Work out the finished part from the listing and answer in its coordinate system (mm). Face numbers are marked on the shaded views. A direction names the side the tool comes from. Round coordinates to 2 decimals unless told otherwise and drop trailing zeros. Write each loop counter-clockwise with the first axis right and the second up, starting at its lowest first coordinate (ties: lowest second). Pieces come first, ordered by that corner, then holes. Notation, with made-up numbers: (87, 16.5) -> (94, 16.5) arc R32 ccw to (94, 52.5) -> close; hole circle Ø9 at (74, -34.75). An arc over 180 degrees is marked (long way). One line per item, written item: value.
```python
from build123d import *

# Parameters (mm, degrees)
SKETCH2_W               = 90
SKETCH2_H               = 90
BOSS_EXTRUDE1_DEPTH     = 103
SKETCH4_W               = 24
SKETCH4_H               = 25
SKETCH4_W_2             = 40
SKETCH4_H_2             = 17.5
SKETCH4_W_3             = 3
SKETCH4_H_3             = 4
SKETCH5_R               = 10
CUT_EXTRUDE1_DEPTH      = 46
CUT_EXTRUDE1_DEPTH_BACK = 46
SKETCH6_W               = 80.499612835
SKETCH6_H               = 43.101198191
CUT_EXTRUDE2_DEPTH      = 46
CUT_EXTRUDE2_DEPTH_BACK = 46
CUT_EXTRUDE3_DEPTH      = 103
CUT_EXTRUDE4_REACH      = 92
SKETCH10_R              = 1.75
FILLET1_R               = 1


with BuildPart() as part:
    # Sketch2 → Boss-Extrude1 (new body)
    with BuildSketch(Plane.XY):
        Rectangle(SKETCH2_W, SKETCH2_H)
    extrude(amount=BOSS_EXTRUDE1_DEPTH)

    # Sketch4 → Cut-Revolve2 (revolve, cut)
    with BuildSketch(Plane(origin=(0, 0, 0), x_dir=(1, 0, 0), z_dir=(0, 1, 0))):
        with Locations((12, -12.5)):
            Rectangle(SKETCH4_W, SKETCH4_H)
        Polygon((0, -25), (0, -39.420654857), (24, -25), align=None)
        with Locations((50, -8.75)):
            Rectangle(SKETCH4_W_2, SKETCH4_H_2)
        with Locations((28.5, -4.5)):
            Rectangle(SKETCH4_W_3, SKETCH4_H_3)
    revolve(axis=Axis((0, 0, 0), (0, 0, 1)), mode=Mode.SUBTRACT)

    # Sketch5 → Cut-Extrude1 (cut, two sides)
    with BuildSketch(Plane(origin=(0, 0, 0), x_dir=(0, 0, -1), z_dir=(1, 0, 0))) as cut_extrude1_sk:
        with Locations((-77.5, 0)):
            Circle(SKETCH5_R)
    extrude(amount=CUT_EXTRUDE1_DEPTH, mode=Mode.SUBTRACT)
    extrude(cut_extrude1_sk.sketch, amount=-CUT_EXTRUDE1_DEPTH_BACK, mode=Mode.SUBTRACT)

    # Sketch6 → Cut-Revolve3 (revolve, cut)
    with BuildSketch(Plane(origin=(0, 0, 0), x_dir=(0, 0, -1), z_dir=(1, 0, 0))):
        with Locations((-94.419607416, 51.550599096)):
            Rectangle(SKETCH6_W, SKETCH6_H)
    revolve(axis=Axis((0, 0, 0), (0, 0, 1)), mode=Mode.SUBTRACT)

    # Sketch7 → Cut-Extrude2 (cut, two sides)
    with BuildSketch(Plane(origin=(0, 0, 0), x_dir=(0, 0, -1), z_dir=(1, 0, 0))) as cut_extrude2_sk:
        with BuildLine():
            Line((-103, 30), (-103, 0))
            ThreePointArc((-103, 0), (-95.748626332, 19.557607216), (-77.5, 29.6605799))
            Line((-77.5, 29.6605799), (-77.5, 30))
            Line((-77.5, 30), (-103, 30))
        make_face()
        with BuildLine():
            ThreePointArc((-77.5, -29.6605799), (-95.748626332, -19.557607216), (-103, 0))
            Line((-103, 0), (-103, -30))
            Line((-103, -30), (-77.5, -30))
            Line((-77.5, -30), (-77.5, -29.6605799))
        make_face()
    extrude(amount=CUT_EXTRUDE2_DEPTH, mode=Mode.SUBTRACT)
    extrude(cut_extrude2_sk.sketch, amount=-CUT_EXTRUDE2_DEPTH_BACK, mode=Mode.SUBTRACT)

    # Sketch8 → Cut-Extrude3 (cut)
    with BuildSketch(Plane.XY.offset(54.169800998)):
        with BuildLine():
            ThreePointArc((30, 0), (28.722813233, 8.660254038), (25, 16.583123952))
            Line((25, 16.583123952), (25, -16.583123952))
            ThreePointArc((25, -16.583123952), (28.722813233, -8.660254038), (30, 0))
        make_face()
        with BuildLine():
            Line((-25, -16.583123952), (-25, 16.583123952))
            ThreePointArc((-25, 16.583123952), (-30, 0), (-25, -16.583123952))
        make_face()
        with BuildLine():
            ThreePointArc((10, 28.284271247), (0, 30), (-10, 28.284271247))
            Line((-10, 28.284271247), (-10, -28.284271247))
            ThreePointArc((-10, -28.284271247), (0, -30), (10, -28.284271247))
            Line((10, -28.284271247), (10, 28.284271247))
        make_face()
    extrude(amount=CUT_EXTRUDE3_DEPTH, mode=Mode.SUBTRACT)

    # Sketch10 → Cut-Extrude4 (cut, up to next)
    with BuildSketch(Plane(origin=(0, 45, 0), x_dir=(1, 0, 0), z_dir=(0, 1, 0)), mode=Mode.PRIVATE) as cut_extrude4_sk1:
        with Locations((0, -32.5)):
            Circle(SKETCH10_R)
    cut_extrude4_tool1 = extrude(cut_extrude4_sk1.sketch, amount=-CUT_EXTRUDE4_REACH, mode=Mode.PRIVATE) & part.part
    add(cut_extrude4_tool1.solids().sort_by_distance((0, 45, 32.5))[0], mode=Mode.SUBTRACT)

    # Fillet1
    fillet1_edges = [part.edges().sort_by_distance(p)[0] for p in [
        (18.452078799, 23.654191764, 54.169800998),
        (18.452078799, -23.654191764, 54.169800998),
        (-18.452078799, -23.654191764, 54.169800998),
        (25, 0, 54.169800998),
        (-25, 0, 54.169800998),
        (-10, 0, 54.169800998),
        (10, 0, 54.169800998),
        (-30, 0, 17.5),
        (-18.452078799, 23.654191764, 54.169800998),
    ]]
    fillet(fillet1_edges, radius=FILLET1_R)


solid = part.part
```
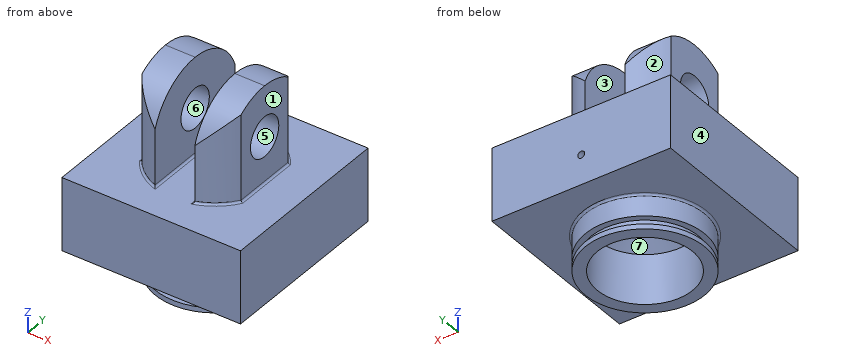
(1) Find section B-B on z = 90.5. Give the vertices of the cut face in (x, y), plus the area to 3 significant figures.
Reported:
outline: (-25, -16.58) arc R30 ccw to (-17.5, -24.37) -> (-10, -24.37) -> (-10, 24.37) -> (-17.5, 24.37) arc R30 ccw to (-25, 16.58) -> close; (10, -24.37) -> (17.5, -24.37) arc R30 ccw to (25, -16.58) -> (25, 16.58) arc R30 ccw to (17.5, 24.37) -> (10, 24.37) -> close
area: 1,360 mm2
(2) Find section D-D on y = -5.5. Give the number of separate pieces and of enclosed holes in the cut face, plus the area to 3 significant figures.
Reported:
separate pieces: 3
enclosed holes: 0
area: 3,790 mm2
(3) For a pull along Z with two mould halves and no side action, classify the marked faces 4, 5, 6 and 7 as pulls with the +Z half, pulls with the -Z half, needs draft (parallel to the pull), parting line crosses it, or undercut.
Reported:
face 4: needs draft
face 5: undercut
face 6: undercut
face 7: pulls with the -Z half
(4) Consider probe 1 along X at (y, z) = (19, 32.5); probe 2 along Y at (x, z) = (0, 5); probe 3 along X at (y, z) = (8, 69.5). Determine where each line is inside the solid, lowest interval first.
Reported:
probe 1: x = -45 to -1.75, 1.75 to 45
probe 2: y = -27 to -24, 24 to 27
probe 3: x = -25 to -10, 10 to 25
(5) A tool of negligible diameter and unlimited length cuts with its end or side. For the marked faces 1, 2 and 3, from which of +Z, -Z, +X, -X, +Y, -Y can it reach the whole face along a straight path? Write none if from no direction.
Reported:
face 1: +Z, +X, +Y, -Y
face 2: +Z, -X, +Y
face 3: +Z, +Y, -Y
(6) Find section C-C on z = 20.5. Give the vertices of the cut face in (x, y), plus the area to 3 significant figures.
Reported:
outline: (-45, -45) -> (45, -45) -> (45, 45) -> (-45, 45) -> close; hole circle Ø48 at (0, 0)
area: 6,290 mm2
(7) Find section A-A on z = 77.5. Give the vertices of the cut face in (x, y), plus the area to 3 significant figures.
Reported:
outline: (-25, -16.58) arc R30 ccw to (-10, -28.28) -> (-10, -10) -> (-25, -10) -> close; (-25, 10) -> (-10, 10) -> (-10, 28.28) arc R30 ccw to (-25, 16.58) -> close; (10, -28.28) arc R30 ccw to (25, -16.58) -> (25, -10) -> (10, -10) -> close; (10, 10) -> (25, 10) -> (25, 16.58) arc R30 ccw to (10, 28.28) -> close
area: 825 mm2
(8) Flat-ended cylindrical pins translate along their axes: pin 1 Ø3 at (x, y) = (-10.5, -34) entering from +Z; pin 2 Ø8 at (x, y) = (-22.5, 13.5) entering from +Z; pin 3 Ø2 at (x, z) = (0, 32.5) entering from +Y. Find the tip coordinate at first contact, or state that the pin passes through.
Reported:
pin 1: stops at z = 54.17
pin 2: stops at z = 101.46
pin 3: stops at y = -9.85
